The model under review builds one solid part; all positions refer to its coordinate system, in mm. A direction names the side the tool comes from. Round coordinates to 2 decimals unless told otherwise and drop trailing zeros. Write each loop counter-clockwise with the first axis right and the second up, starting at its lowest first coordinate (ties: lowest second). Pieces come first, ordered by that corner, then holes. Notation, with made-up numbers: (77.5, -27) -> (102.5, -27) arc R16 cw to (102.5, -22) -> close; hole circle Ø2 at (17, 40). An arc over 180 degrees is marked (long way). Answer as a JSON object with one key per item and string values. Group by question number.
1) We need section B-B, the plane z = 1. Write out the cut boundary in (x, y), then the cut area to 3 significant figures.
2) Insertion check: pin 1 Ø7 at (x, z) = (3.5, 6.5) entering from +Y; pin 2 Ø10.5 at (x, y) = (24.75, 11.25) entering from +Z; pin 3 Ø1.6 at (x, z) = (22.5, 1) entering from -Y. Each pin has a flat end and moves straight along its axis. Give the tip position at first contact, or say it passes through.
3) We need section C-C, the plane x = 29.5. Write out the cut boundary in (y, z), then the cut area to 3 significant figures.
4) We need section D-D, the plane z = 14. Write out the cut boundary in (x, y).
5) To check wall thickness, follow probe 1 along Z at (x, y) = (29.5, -1.3); probe 2 along Z at (x, y) = (3, 12.25); probe 3 along Y at (x, z) = (7, 17.5). State the ranges of each line that lie inside material, in increasing order. Write a range as [from, to].
6) Machinability: for faces 4 (the flat face through (23, 0, 1)), 5 (the flat face through (34, -0.3, 5.1)), 6 (the flat face through (29, 0, 10)), which of the approach directions +Z, -Z, +X, -X, +Y, -Y give a long, thin tool a straight path to every point of the face, cutting with its end or side? Answer none if there is none.
7) We need section A-A, the plane y = 1.5. Write out the cut boundary in (x, z).
8) Mouldability with a two-part tool opening along Z and no side actions: class faces 1 (the flat face through (0, -0.3, 5.1)), 2 (the cylindrical face through (28, -1, 14)), 3 (the flat face through (4, -1, 18.5)) as pulls with the +Z half, pulls with the -Z half, needs draft (parallel to the pull), parting line crosses it, or undercut.
from build123d import *

# Parameters (mm, degrees)
BOX_W           = 34
BOX_H           = 17
BOX_DEPTH       = 2
SKETCH_R        = 3.25
POCKET_DEPTH    = 2
SKETCH001_W     = 6.498788
SKETCH001_H     = 3.187234
POCKET001_DEPTH = 2
SKETCH002_W     = 9
SKETCH002_H     = 2
PAD_DEPTH       = 2
SKETCH003_W     = 9
SKETCH003_H     = 2
PAD001_DEPTH    = 16.5
SKETCH004_R     = 1.5
POCKET002_DEPTH = 2


with BuildPart() as part:
    # Box → Box (new body)
    with BuildSketch(Plane.XY):
        with Locations((17, 8.5)):
            Rectangle(BOX_W, BOX_H)
    extrude(amount=BOX_DEPTH)

    # Sketch → Pocket (cut)
    with BuildSketch(Plane.XY.offset(2)):
        with Locations((9.25, 11.25)):
            Circle(SKETCH_R)
        with Locations((24.75, 11.25)):
            Circle(SKETCH_R)
        with Locations((17, 3.25)):
            Circle(SKETCH_R)
    extrude(amount=-POCKET_DEPTH, mode=Mode.SUBTRACT)

    # Sketch001 → Pocket001 (cut)
    with BuildSketch(Plane.XY.offset(2)):
        with Locations((17, 1.593617)):
            Rectangle(SKETCH001_W, SKETCH001_H)
    extrude(amount=-POCKET001_DEPTH, mode=Mode.SUBTRACT)

    # Sketch002 → Pad (new body)
    with BuildSketch(Plane.XZ):
        with Locations((4.5, 1)):
            Rectangle(SKETCH002_W, SKETCH002_H)
        with Locations((29.5, 1)):
            Rectangle(SKETCH002_W, SKETCH002_H)
    extrude(amount=PAD_DEPTH)

    # Sketch003 → Pad001 (new body)
    with BuildSketch(Plane.XY.offset(2)):
        with Locations((4.5, -1)):
            Rectangle(SKETCH003_W, SKETCH003_H)
        with Locations((29.5, -1)):
            Rectangle(SKETCH003_W, SKETCH003_H)
    extrude(amount=PAD001_DEPTH)

    # Sketch004 → Pocket002 (cut)
    with BuildSketch(Plane.XZ.offset(2)):
        with Locations((4.5, 14)):
            Circle(SKETCH004_R)
        with Locations((29.5, 14)):
            Circle(SKETCH004_R)
    extrude(amount=-POCKET002_DEPTH, mode=Mode.SUBTRACT)


solid = part.part
Here are the results:
{
 "1": {"outline": "(0, -2) -> (9, -2) -> (9, 0) -> (13.75, 0) -> (13.75, 3.19) arc R3.25 cw (long way) to (20.25, 3.19) -> (20.25, 0) -> (25, 0) -> (25, -2) -> (34, -2) -> (34, 17) -> (0, 17) -> close; hole circle Ø6.5 at (9.25, 11.25); hole circle Ø6.5 at (24.75, 11.25)", "area": "510 mm^2"},
 "2": {"pin 1": "stops at y = 0", "pin 2": "stops at z = 2", "pin 3": "stops at y = 0"},
 "3": {"outline": "(-2, 0) -> (17, 0) -> (17, 2) -> (0, 2) -> (0, 12.5) -> (-2, 12.5) -> close; (-2, 15.5) -> (0, 15.5) -> (0, 18.5) -> (-2, 18.5) -> close", "area": "65.0 mm^2"},
 "4": {"outline": "(0, -2) -> (3, -2) -> (3, 0) -> (0, 0) -> close; (6, -2) -> (9, -2) -> (9, 0) -> (6, 0) -> close; (25, -2) -> (28, -2) -> (28, 0) -> (25, 0) -> close; (31, -2) -> (34, -2) -> (34, 0) -> (31, 0) -> close"},
 "5": {"probe 1": "z = [0, 12.5], [15.5, 18.5]", "probe 2": "z = [0, 2]", "probe 3": "y = [-2, 0]"},
 "6": {"face 4": "+Z, -Z, -Y", "face 5": "+Z, -Z, +X, +Y, -Y", "face 6": "+Z, +X, -X, +Y"},
 "7": {"outline": "(0, 0) -> (13.75, 0) -> (13.75, 2) -> (0, 2) -> close; (20.25, 0) -> (34, 0) -> (34, 2) -> (20.25, 2) -> close"},
 "8": {"face 1": "needs draft", "face 2": "undercut", "face 3": "pulls with the +Z half"}
}
